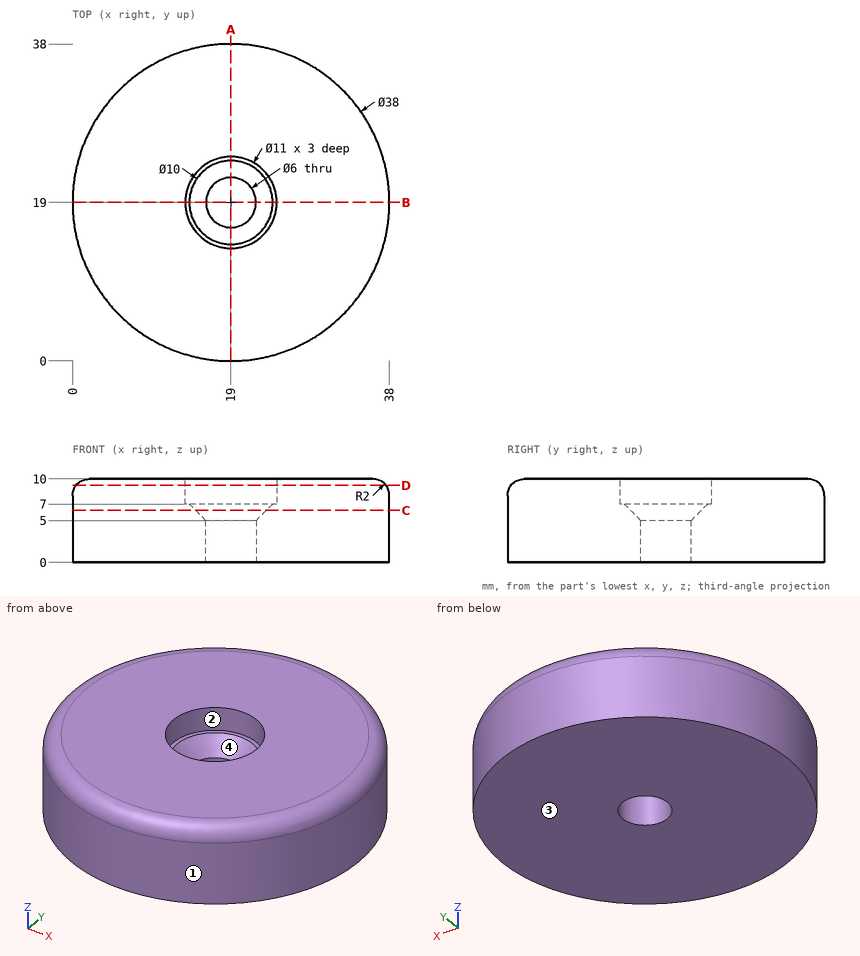
The drawing under review shows one solid part. Ordinate dimensions are in mm from its lowest x, y, z. Coordinates: 2 decimals unless noted, no trailing zeros. Write each loop counter-clockwise with the first axis right and the second up, starting at its lowest first coordinate (ties: lowest second). Pieces come first, ordered by that corner, then holes. Notation, with made-up numbers: (75.25, 2.5) - (86.25, 2.5) arc R26 cw to (86.25, 40.5) - close; hole circle Ø10 at (-34.75, -38). An arc over 180 degrees is marked (long way). Answer in a Markdown table with one row per item. Add a question column.
Q1. We need section C-C, the plane z = 6.25. State the section outline as (x, y) points.
Q2. We need section D-D, the plane z = 9.25. State the section outline as (x, y) points, and give its area (3 significant figures).
Q3. Draft analysis for pull direction X (two halves, no side actions). For the marked faces 1, 2, 3 and 4, state which applies: +X half, -X half, draft (parallel to the pull), parting line (faces both ways), or undercut.
Q4. For P1, Ø1, axis at x = 21, z = 9, coming from the +Y side; P2, Ø1, axis at x = 7.5, z = 1, coming from the -Y side; P3, Ø2, axis at y = 16.5, z = 1.5, coming from the -X side, all flat-tipped, find the tip position at first contact; note any pin that passes through.
Q5. We need section A-A, the plane x = 19. State the section outline as (y, z) points.
Q6. For probe 1 along Y at (x, z) = (19, 8.1); probe 2 along Y at (x, z) = (19, 1.5); probe 3 along Y at (x, z) = (10.5, 1), list the stretches that pass through material, from the lowest coordinate up.
Answer list:
| question | item | result |
|---|---|---|
| 1 | outline | circle Ø38 at (19, 19); hole circle Ø8.5 at (19, 19) |
| 2 | outline | circle Ø37.12 at (19, 19); hole circle Ø11 at (19, 19) |
| 2 | area | 987 mm2 |
| 3 | face 1 | parting line |
| 3 | face 2 | undercut |
| 3 | face 3 | draft |
| 3 | face 4 | undercut |
| 4 | P1 | stops at y = 37.84 |
| 4 | P2 | stops at y = 3.51 |
| 4 | P3 | stops at x = 0.06 |
| 5 | outline | (0, 0) - (16, 0) - (16, 5) - (14, 7) - (13.5, 7) - (13.5, 10) - (2, 10) arc R2 ccw to (0, 8) - close; (22, 0) - (38, 0) - (38, 8) arc R2 ccw to (36, 10) - (24.5, 10) - (24.5, 7) - (24, 7) - (22, 5) - close |
| 6 | probe 1 | y = 0 to 13.5, 24.5 to 38 |
| 6 | probe 2 | y = 0 to 16, 22 to 38 |
| 6 | probe 3 | y = 2.01 to 35.99 |
